Read the model definition and answer for the solid it produces. Units are mm, in the model's axes. A direction names the side the tool comes from. Coordinates: 2 decimals unless noted, no trailing zeros. Loops run counter-clockwise (first coordinate to the right, second up) from the corner with the lowest first, then second, coordinate; pieces in that order, holes last. Notation, with made-up numbers: (84, 35) -> (97, 35) arc R17 cw to (97, 46) -> close; hole circle Ø11 at (58.25, -13.75). An arc over 180 degrees is marked (long way). One line per question, with ' | ' between items. Start each with the question number.
```python
from build123d import *

# Parameters (mm, degrees)
ESQUISSE1_R             = 54.5
ESQUISSE1_R_2           = 47.5
BOSS_EXTRU_1_DEPTH      = 15
ESQUISSE2_W             = 1
ESQUISSE2_H             = 10.244333075
ENL_V_MAT_EXTRU_1_DEPTH = 6


with BuildPart() as part:
    # Esquisse1 → Boss.-Extru.1 (new body)
    with BuildSketch(Plane.XY):
        Circle(ESQUISSE1_R)
        Circle(ESQUISSE1_R_2, mode=Mode.SUBTRACT)
    extrude(amount=BOSS_EXTRU_1_DEPTH)

    # Esquisse2 → Enlèv. mat.-Extru.1 (cut)
    with BuildSketch(Plane(origin=(0, 0, 0), x_dir=(-1, 0, 0), z_dir=(0, 0, -1))):
        Polygon((48.965976814, 27.693169625), (40.094124126, 22.571003088), (39.594124126, 23.437028491), (48.465976814, 28.559195029), align=None)
        with Locations((0, 51.130198117)):
            Rectangle(ESQUISSE2_W, ESQUISSE2_H)
        Polygon((48.465976814, -28.559195029), (39.594124126, -23.437028491), (40.094124126, -22.571003088), (48.965976814, -27.693169625), align=None)
        with Locations((0, -51.130198117)):
            Rectangle(ESQUISSE2_W, ESQUISSE2_H)
        Polygon((-48.965976814, -27.693169625), (-40.094124126, -22.571003088), (-39.594124126, -23.437028491), (-48.465976814, -28.559195029), align=None)
        Polygon((-48.465976814, 28.559195029), (-39.594124126, 23.437028491), (-40.094124126, 22.571003088), (-48.965976814, 27.693169625), align=None)
    extrude(amount=-ENL_V_MAT_EXTRU_1_DEPTH, mode=Mode.SUBTRACT)


solid = part.part
```
(1) Determine the mould class of faces 4 (the flat face through (-43.873, 25.907, 2.958)), 5 (the flat face through (-44.37, -25.04, 2.96)), 6 (the flat face through (-0.5, -51, 3)) for opening direction Y: +Y half, -Y half, draft (parallel to the pull), parting line (faces both ways), or undercut.
(2) Each of these flat-tipped pins is pushed along its axis until it touches: pin 1 Ø8 at (y, z) = (-34, 7.5) entering from -X; pin 2 Ø1.8 at (y, z) = (51, 3.5) entering from -X; pin 3 Ø1.8 at (y, z) = (-50, 3.5) entering from +X. Where does it stop, or does it pass through?
(3) Section C-C on z = 8.5 is taken. Write down the section's boundary in (x, y).
(4) Find the intervals of material crossed by probe 1 along Y at (x, z) = (0, 11); probe 2 along Y at (x, z) = (-28, 9.25), in increasing order. Write a range as from..to.
(5) Section B-B on x = 31.5 is taken. Write down the section's boundary in (y, z), plus the area to 3 significant figures.
(6) Section A-A on y = 0 is taken. Write down the section's boundary in (x, z), plus the area to 3 significant figures.
(7) A tool of negligible diameter and unlimited length cuts with its end or side. For faces 1 (the cylindrical face through (-10.3, -46.37, 7.4)), 2 (the flat face through (-44.46, 25.09, 2.96)), 3 (the flat face through (-0.5, 51, 3)), from which of +Z, -Z, +X, -X, +Y, -Y can it reach the whole face along a straight path? Write none if from no direction.
Working result:
1) face 4: undercut | face 5: undercut | face 6: draft
2) pin 1: stops at x = -45.5 | pin 2: stops at x = -21.45 | pin 3: stops at x = 23.65
3) outline: circle Ø109 at (0, 0); hole circle Ø95 at (0, 0)
4) probe 1: y = -54.5..-47.5, 47.5..54.5 | probe 2: y = -46.76..-38.37, 38.37..46.76
5) outline: (-44.47, 0) -> (-35.55, 0) -> (-35.55, 15) -> (-44.47, 15) -> close; (35.55, 0) -> (44.47, 0) -> (44.47, 15) -> (35.55, 15) -> close | area: 268 mm2
6) outline: (-54.5, 0) -> (-47.5, 0) -> (-47.5, 15) -> (-54.5, 15) -> close; (47.5, 0) -> (54.5, 0) -> (54.5, 15) -> (47.5, 15) -> close | area: 210 mm2
7) face 1: +Z, -Z | face 2: -Z | face 3: -Z, +Y, -Y
